Solid Edge part; units mm, degrees
sketch "Sketch1" plane through (0, 0, 0) normal (0, -1, 0) x (1, 0, 0)
  line L0 (4, 22) -> (4, 4)
  line L1 (4, 4) -> (22, 4)
  line L2 (22, 4) -> (22, 0)
  line L3 (22, 0) -> (0, 0)
  line L4 (0, 0) -> (0, 22)
  line L5 (0, 22) -> (4, 22)
extrude "Protrusion1" add sketch "Sketch1" against normal blind 18
hole "Agujero_1" at (13, 9, 4) direction (0, 0, -1) diameter 4 end up to next
hole "Agujero_2" at (4, 9, 13) direction (-1, 0, 0) diameter 4 end up to next
sketch "Sketch2" plane through (11, 0, 11) normal (0, -1, 0) x (1, 0, 0)
  line L0 (-7, 2) -> (2, -7)
  line L1 (2, -7) -> (-7, -7)
  line L2 (-7, -7) -> (-7, 2)
extrude "ProtrusiónExtruida_2" add sketch "Sketch2" against normal blind 3
mirror "Mirror1" about plane through (11, 9, 11) normal (0, -1, 0) of "ProtrusiónExtruida_2"
fillet "Redondeo_2" radius 6 4 edges at (2, 0, 22) (2, 18, 22) (22, 18, 2) (22, 0, 2)
chamfer "Chaflán_1" distance 2.3 angle 45 2 edges at (11, 9, 4) (4, 7, 13)
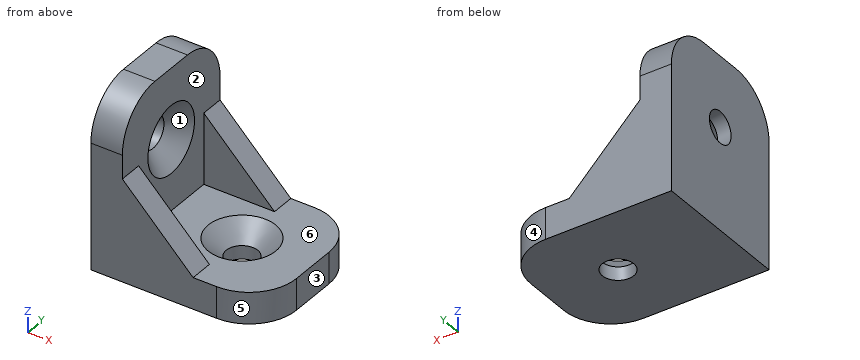
Build history of the part. All positions in model axes, mm. Face numbers are marked on the shaded views. A direction names the side the tool comes from. Round coordinates to 2 decimals unless told otherwise and drop trailing zeros. Order: outer loops, then holes, each group sorted by start corner. A loop starts at its lowest first (then second) coordinate and runs counter-clockwise, first axis right, second up. Notation, with made-up numbers: (80.25, 53) - (110.25, 53) arc R37 ccw to (110.25, 91) - close; hole circle Ø6 at (41, 51.25). An arc over 180 degrees is marked (long way). Use a Markdown table: item, result.
1) Pull direction Y, two halves, no side cores. Call the marked faces 1, 2, 3 and 4: pulls with the +Y half, pulls with the -Y half, needs draft (parallel to the pull), parting line crosses it, or undercut.
Recorded:
| item | result |
|---|---|
| face 1 | undercut |
| face 2 | undercut |
| face 3 | needs draft |
| face 4 | pulls with the +Y half |
2) Flat gauge pins, fed straight in: pin 1 Ø4.5 at (y, z) = (9, 13) entering from +X; pin 2 Ø4 at (x, z) = (5, 7) entering from -Y; pin 3 Ø5 at (x, y) = (13, 9) entering from +Z; pin 4 Ø9 at (y, z) = (8, 9.5) entering from +X. Where does each tip first touch, or does it go through?
Recorded:
| item | result |
|---|---|
| pin 1 | stops at x = 1.95 |
| pin 2 | stops at y = 0 |
| pin 3 | stops at z = 2.2 |
| pin 4 | stops at x = 4 |
3) Saw through at B-B on x = 3.25. Write the cut outline in (y, z).
Recorded:
| item | result |
|---|---|
| outline | (0, 0) - (18, 0) - (18, 16) arc R6 ccw to (12, 22) - (6, 22) arc R6 ccw to (0, 16) - close; hole circle Ø7.1 at (9, 13) |
4) Tool access for the marked faces 5 and 6: list every direction of +Z, -Z, +X, -X, +Y, -Y with a clear straight run to the whole face (end or side of a thin tool).
Recorded:
| item | result |
|---|---|
| face 5 | +Z, -Z, +X, -Y |
| face 6 | +Z, +X |
5) Wall check: L1, parallel to Z at x = 0.8, y = 9; L2, parallel to Y at x = 0.65, z = 13. Give the ranges that are in metal, low to high.
Recorded:
| item | result |
|---|---|
| L1 | z = 0 to 11, 15 to 22 |
| L2 | y = 0 to 7, 11 to 18 |
6) Saw through at C-C on z = 4.5. Write the cut outline in (x, y).
Recorded:
| item | result |
|---|---|
| outline | (0, 0) - (12.5, 0) - (12.5, 3) - (4, 3) - (4, 15) - (12.5, 15) - (12.5, 18) - (0, 18) - close |
7) Saw through at D-D on y = 14. Write the cut outline in (x, z), and give its area (3 significant figures).
Recorded:
| item | result |
|---|---|
| outline | (0, 0) - (21.66, 0) - (21.66, 4) - (4, 4) - (4, 21.66) - (0, 21.66) - close |
| area | 157 mm² |
8) Saw through at A-A on y = 9. Write the cut outline in (x, z), and give its area (3 significant figures).
Recorded:
| item | result |
|---|---|
| outline | (0, 0) - (11, 0) - (11, 1.7) - (8.7, 4) - (4, 4) - (4, 8.7) - (1.7, 11) - (0, 11) - close; (0, 15) - (1.7, 15) - (4, 17.3) - (4, 22) - (0, 22) - close; (15, 0) - (22, 0) - (22, 4) - (17.3, 4) - (15, 1.7) - close |
| area | 117 mm² |
